from build123d import *

# Parameters (mm, degrees)
SKETCH1_W           = 22.8
SKETCH1_H           = 12.3
BOSS_EXTRUDE1_DEPTH = 2
SKETCH2_W           = 32.8
SKETCH2_H           = 17.3
SKETCH2_W_2         = 22.8
SKETCH2_H_2         = 12.3
BOSS_EXTRUDE2_DEPTH = 20.2
SKETCH3_W           = 15.2
SKETCH3_H           = 11.3
CUT_EXTRUDE1_DEPTH  = 5
FILLET1_R           = 1
SKETCH4_R           = 0.75
CUT_EXTRUDE2_DEPTH  = 5
SKETCH5_W           = 3.5
SKETCH5_H           = 17.3
CUT_EXTRUDE3_DEPTH  = 28.419381831
FILLET2_R           = 1
SKETCH8_W           = 14.2
SKETCH8_H           = 8
BOSS_EXTRUDE4_DEPTH = 3
SKETCH9_R           = 1.75
CUT_EXTRUDE5_DEPTH  = 37.057627487
FILLET4_R           = 2
SKETCH10_W          = 2.29579642
SKETCH10_H          = 17.3
CUT_EXTRUDE6_DEPTH  = 31.890492065
FILLET5_R           = 1
FILLET6_R           = 1


with BuildPart() as part:
    # Sketch1 → Boss-Extrude1 (new body)
    with BuildSketch(Plane.XY):
        Rectangle(SKETCH1_W, SKETCH1_H)
    extrude(amount=BOSS_EXTRUDE1_DEPTH)

    # Sketch2 → Boss-Extrude2 (add)
    with BuildSketch(Plane.XY.offset(2)):
        Rectangle(SKETCH2_W, SKETCH2_H)
        Rectangle(SKETCH2_W_2, SKETCH2_H_2, mode=Mode.SUBTRACT)
    extrude(amount=-BOSS_EXTRUDE2_DEPTH)

    # Sketch3 → Cut-Extrude1 (cut)
    with BuildSketch(Plane.ZY.offset(16.4)):
        with Locations((-10.6, 0)):
            Rectangle(SKETCH3_W, SKETCH3_H)
    extrude(amount=-CUT_EXTRUDE1_DEPTH, mode=Mode.SUBTRACT)

    # Fillet1
    fillet1_edges = [part.edges().sort_by_distance(p)[0] for p in [
        (-13.9, 5.65, -3),
        (-13.9, -5.65, -3),
    ]]
    fillet(fillet1_edges, radius=FILLET1_R)

    # Sketch4 → Cut-Extrude2 (cut)
    with BuildSketch(Plane(origin=(0, 0, -18.2), x_dir=(-1, 0, 0), z_dir=(0, 0, -1))):
        with Locations((-13.75, 0)):
            Circle(SKETCH4_R)
    extrude(amount=-CUT_EXTRUDE2_DEPTH, mode=Mode.SUBTRACT)

    # Sketch5 → Cut-Extrude3 (cut, through all)
    with BuildSketch(Plane(origin=(0, 0, -18.2), x_dir=(-1, 0, 0), z_dir=(0, 0, -1))):
        with Locations((14.65, 0)):
            Rectangle(SKETCH5_W, SKETCH5_H)
    extrude(amount=-CUT_EXTRUDE3_DEPTH, mode=Mode.SUBTRACT)

    # Fillet2
    fillet2_edges = [part.edges().sort_by_distance(p)[0] for p in [
        (16.4, 8.65, -8.1),
        (-12.9, 5.357106781, -3.292893219),
        (-12.9, -7.15, -18.2),
        (-12.9, 7.15, -18.2),
        (-12.9, -5.65, -11.1),
        (-12.9, -5.357106781, -3.292893219),
        (-12.9, 0, -3),
        (-12.9, 5.65, -11.1),
        (-12.9, 0, 2),
        (-12.9, -8.65, -8.1),
        (-12.9, 8.65, -8.1),
    ]]
    fillet(fillet2_edges, radius=FILLET2_R)

    # Sketch8 → Boss-Extrude4 (add)
    with BuildSketch(Plane(origin=(16.4, 0, 0), x_dir=(0, 0, -1), z_dir=(1, 0, 0))):
        with Locations((8.1, -12.65)):
            Rectangle(SKETCH8_W, SKETCH8_H)
    extrude(amount=-BOSS_EXTRUDE4_DEPTH)

    # Sketch9 → Cut-Extrude5 (cut, through all)
    with BuildSketch(Plane.ZY.offset(-13.4)):
        with Locations((-10.7, -12.65)):
            Circle(SKETCH9_R)
        with Locations((-5.5, -12.65)):
            Circle(SKETCH9_R)
    extrude(amount=-CUT_EXTRUDE5_DEPTH, mode=Mode.SUBTRACT)

    # Fillet4
    fillet4_edges = [part.edges().sort_by_distance(p)[0] for p in [
        (14.9, -16.65, -1),
        (14.9, -8.65, -1),
        (14.9, -8.65, -15.2),
        (14.9, -16.65, -15.2),
    ]]
    fillet(fillet4_edges, radius=FILLET4_R)

    # Sketch10 → Cut-Extrude6 (cut, through all)
    with BuildSketch(Plane(origin=(0, 0, -18.2), x_dir=(-1, 0, 0), z_dir=(0, 0, -1))):
        with Locations((12.54789821, 0)):
            Rectangle(SKETCH10_W, SKETCH10_H)
    extrude(amount=-CUT_EXTRUDE6_DEPTH, mode=Mode.SUBTRACT)

    # Fillet5
    fillet5_edges = [part.edges().sort_by_distance(p)[0] for p in [
        (16.4, -0.5, 2),
        (16.107106781, 8.357106781, 2),
        (-11.4, 6.15, -9.1),
        (-11.4, 7.4, -18.2),
        (-11.4, 8.65, -8.1),
        (-11.4, 0, 2),
        (-11.4, -8.65, -8.1),
        (-11.4, -7.4, -18.2),
        (-11.4, -6.15, -9.1),
        (-11.4, 0, 0),
        (2.5, -8.65, 2),
        (2, 8.65, 2),
    ]]
    fillet(fillet5_edges, radius=FILLET5_R - 0.0001)  # a hair under: the kernel refuses the full size

    # Fillet6
    fillet6_edges = [part.edges().sort_by_distance(p)[0] for p in [
        (13.4, -8.65, -8.1),
    ]]
    fillet(fillet6_edges, radius=FILLET6_R)


solid = part.part
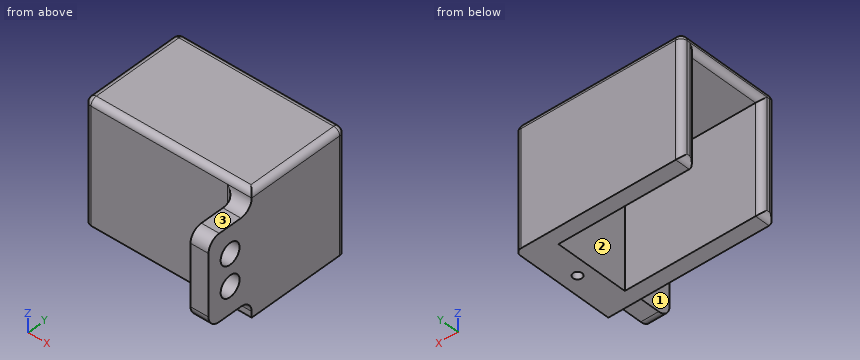
Verification items for the finished model (mm, model axes). Face numbers are marked on the shaded views. A direction names the side the tool comes from. Round coordinates to 2 decimals unless told otherwise and drop trailing zeros. Loops run counter-clockwise (first coordinate to the right, second up) from the corner with the lowest first, then second, coordinate; pieces in that order, holes last. Notation, with made-up numbers: M 17.25,85 L 39.25,85 A22 ccw 39.25,112 Z; hole C 14.25,-26 d11. An arc over 180 degrees is marked long. Write each question's results on one line, items separated by ' | '.
1) Section check A-A on z = -10.7. Record the boundary of the cut face in (x, y), then the cut area to 3 significant figures.
Checks:
outline: M -11.4,-7.65 A1 ccw -10.4,-8.65 L 12.4,-8.65 A1 cw 13.4,-9.65 L 13.4,-10.9 L 16.4,-10.9 L 16.4,7.65 A1 ccw 15.4,8.65 L -10.4,8.65 A1 ccw -11.4,7.65 L -11.4,7.15 A1 ccw -10.4,6.15 L 11.4,6.15 L 11.4,-6.15 L -10.4,-6.15 A1 ccw -11.4,-7.15 Z; M 13.4,-16.65 L 16.4,-16.65 L 16.4,-14.4 L 13.4,-14.4 Z | area: 213 mm2
2) Scan lines: L1, parallel to Y at x = 15.3, z = -10.7; L2, parallel to Y at x = -9, z = -6.75; L3, parallel to X at y = 0, z = -12.25. Record each from-to range of solid material in increasing order. Write a range as from..to.
Checks:
L1: y = -16.65..-14.4, -10.9..8.65 | L2: y = -8.65..-6.15, 6.15..8.65 | L3: x = 11.4..16.4
3) Section check C-C on y = -12.65. Record the boundary of the cut face in (x, z), then the cut area to 3 significant figures.
Checks:
outline: M 13.4,-15.2 L 16.4,-15.2 L 16.4,-12.45 L 13.4,-12.45 Z; M 13.4,-8.95 L 16.4,-8.95 L 16.4,-7.25 L 13.4,-7.25 Z; M 13.4,-3.75 L 16.4,-3.75 L 16.4,-1 L 13.4,-1 Z | area: 21.6 mm2
4) Gauge pin test, flat ends, axial feed: P1, Ø1, axis at x = 2.5, z = -14.5, coming from the -Y side; P2, Ø0.9, axis at x = 14, y = -12.5, coming from the -Z side; P3, Ø8, axis at x = 12, y = -13, coming from the -Z side; P4, Ø4, axis at x = 1.5, y = -11, coming from the -Z side. Record the tip position at first contact, or that the pin passes through.
Checks:
P1: stops at y = -8.65 | P2: stops at z = -15.2 | P3: stops at z = -15.8 | P4: passes through
5) Access from +Z, -Z, +X, -X, +Y, -Y to the whole of each face (thin tool, end or side, straight path). Record for the marked faces 1, 2 and 3.
Checks:
face 1: +Z, -Z, -X, -Y | face 2: -Z, -X | face 3: +Z, +X, -X, -Y
6) Section check B-B on x = 13.75. State how many separate pieces and enclosed holes the cut face has, then the cut area to 3 significant figures.
Checks:
separate pieces: 1 | enclosed holes: 2 | area: 436 mm2
